The model under review builds one solid part; all positions refer to its coordinate system, in mm. A direction names the side the tool comes from. Coordinates: 2 decimals unless noted, no trailing zeros. Loops run counter-clockwise (first coordinate to the right, second up) from the corner with the lowest first, then second, coordinate; pieces in that order, holes last. Notation, with made-up numbers: (69, 55) - (105, 55) arc R38 ccw to (105, 94) - close; hole circle Ø2 at (21.25, -2). An arc over 180 degrees is marked (long way). Answer in a Markdown table with one row per item. Add a question column.
(1) Machinability: for faces 1 (the cylindrical face through (136.2, 0.9, 2.7)), 2 (the flat face through (76.637, 5, 6)), 3 (the cylindrical face through (136.25, 7.94, 2.72)), 4 (the flat face through (79.905, 4, 6)), which of the approach directions +Z, -Z, +X, -X, +Y, -Y give a long, thin tool a straight path to every point of the face, cutting with its end or side? Answer none if there is none.
(2) We need section A-A on z = 5.25. Write out the cut boundary in (x, y) (3 decimals).
(3) Mouldability with a two-part tool opening along Y and no side actions: class faces 5 (the cylindrical face through (0.95, 7.98, 1.93)), 6 (the flat face through (21, 5, 3.81)), 7 (the cylindrical face through (43.427, 4.185, 6.993)) as +Y half, -Y half, draft (parallel to the pull), parting line (faces both ways), or undercut.
(4) For P1, Ø5.5, axis at x = 127.5, y = 10.5, coming from the +Z side; P2, Ø6, axis at x = 109, y = 4.5, coming from the -Z side; P3, Ø0.5, axis at y = -0.5, z = 1, coming from the -X side; P4, Ø5.5, axis at x = 49.5, z = 5, coming from the +Y side, all flat-tipped, find the tip position at first contact; note any pin that passes through.
(5) For line 1 along X through (y, z) = (0.75, 4.25) (3 decimals); line 2 along Z through (x, y) = (24, 5.75); line 3 along Y through (x, z) = (75.5, 2.5), list the stretches that pass through material, from the lowest coordinate up.
(6) We need section C-C on x = 74.5. Write out the cut boundary in (y, z), plus the area to 3 significant figures.
(7) We need section D-D on y = 1.25. Write out the cut boundary in (x, z) (3 decimals).
(8) We need section B-B on y = 7.75. Write out the cut boundary in (x, z) (3 decimals).
Autodesk Inventor part; units mm, degrees
ref_plane "YZ Plane" through (0, 0, 0) normal (1, 0, 0) x (0, 1, 0)
ref_plane "XZ Plane" through (0, 0, 0) normal (0, 1, 0) x (-1, 0, 0)
ref_plane "XY Plane" through (0, 0, 0) normal (0, 0, 1) x (1, 0, 0)
sketch "Sketch1" plane through (0, 0, 0) normal (0, 0, 1) x (1, 0, 0)
  point P0 (0, 0)
sketch "Sketch2" plane through (0, 0, 0) normal (0, 0, 1) x (1, 0, 0)
  line L0 (0, 0) -> (137.16, 0)
  line L1 (137.16, 0) -> (137.16, 8.89)
  line L2 (137.16, 8.89) -> (0, 8.89)
  line L3 (0, 8.89) -> (0, 0)
  dimension "d0" = 137.16
  dimension "d3" = 8.89
extrude "Extrusion1" add sketch "Sketch2" along normal blind 3.81
sketch "Sketch3" plane through (0, 8.89, 0) normal (0, 1, 0) x (1, 0, 0)
  line L0 (137.16, 0) -> (137.16, -3.81)
  line L1 (137.16, 0) -> (119.5015, 0)
  line L2 (119.5015, 0) -> (119.5015, -1.6003)
  line L3 (119.5015, -1.6003) -> (137.16, -1.6003)
  line L4 (137.16, -1.6003) -> (137.16, 0)
  point P0 (0, 0)
extrude "Extrusion2" add sketch "Sketch3" along normal blind 3.81
sketch "Sketch4" plane through (0, 0, 0) normal (0, -1, 0) x (1, 0, 0)
  line L0 (0, 0) -> (137.16, 0)
  line L1 (119.5015, 1.6003) -> (137.16, 1.6003)
  line L2 (137.16, 0) -> (119.5015, 0)
  line L3 (119.5015, 0) -> (119.5015, 1.6003)
  line L4 (119.5015, 1.6003) -> (137.16, 1.6003)
  line L5 (137.16, 1.6003) -> (137.16, 0)
extrude "Extrusion3" add sketch "Sketch4" along normal blind 3.81
sketch "Sketch6" plane through (0, 0, 3.81) normal (0, 0, 1) x (1, 0, 0)
  line L0 (119.5015, 8.89) -> (0, 8.89)
  line L1 (0, 0) -> (119.5015, 0)
  line L2 (79.905, 8.89) -> (76.6366, 8.89)
  line L3 (76.6366, 8.89) -> (76.6366, 0)
  line L4 (76.6366, 0) -> (79.905, 0)
  line L5 (79.905, 0) -> (79.905, 8.89)
  dimension "d28" = 119.5015
extrude "Extrusion5" add sketch "Sketch6" along normal blind 7.62
sketch "Sketch7" plane through (79.905, 0, 3.81) normal (1, 0, 0) x (0, 0, -1)
  line L0 (-7.62, 0) -> (-7.62, 8.89)
  circle A0 centre (-7.62, 4.445) radius 4.445
  point P0 (3.81, 0)
extrude "Extrusion6" cut sketch "Sketch7" against normal blind 12.7
sketch "Sketch8" plane through (0, 0, 3.81) normal (0, 0, 1) x (1, 0, 0)
  line L0 (0, 0) -> (119.5015, 0)
  line L1 (119.5015, 8.89) -> (0, 8.89)
  line L2 (45.2172, 0) -> (41.5862, 0)
  line L3 (41.5862, 0) -> (41.5862, 8.89)
  line L4 (41.5862, 8.89) -> (45.2172, 8.89)
  line L5 (45.2172, 8.89) -> (45.2172, 0)
extrude "Extrusion7" add sketch "Sketch8" along normal blind 12.7
fillet "Fillet3" radius 3.175 8 edges at (0, 0, 1.905) (0, 8.89, 1.905) (137.16, 0, 2.7052) (137.16, 8.89, 2.7052) (137.16, -3.81, 0.8002) (137.16, 12.7, 0.8002) (119.5015, -3.81, 0.8002) (119.5015, 12.7, 0.8002)
extrude "Extrusion8" cut sketch "Sketch7" against normal through all
sketch "Sketch9" plane through (41.5862, 0, 16.51) normal (-1, 0, 0) x (0, 0, 1)
  circle A0 centre (-1.585, 4.5756) radius 5.8334
  point P0 (-16.51, 0)
extrude "Extrusion9" cut sketch "Sketch9" against normal through all
properties part number "stweet"
Outcome:
| question | item | result |
|---|---|---|
| 1 | face 1 | +Z, +X, -Y |
| 1 | face 2 | +Z, +Y, -Y |
| 1 | face 3 | +Z, +X, +Y |
| 1 | face 4 | +Z, +X, +Y, -Y |
| 2 | outline | (41.586, 0) - (45.217, 0) - (45.217, 8.89) - (41.586, 8.89) - close; (76.637, 0) - (79.905, 0) - (79.905, 8.89) - (76.637, 8.89) - close |
| 3 | face 5 | +Y half |
| 3 | face 6 | draft |
| 3 | face 7 | undercut |
| 4 | P1 | z = 3.81 |
| 4 | P2 | z = 0 |
| 4 | P3 | x = 119.5 |
| 4 | P4 | y = 8.89 |
| 5 | line 1 | 41.586 to 45.217, 76.637 to 79.905 |
| 5 | line 2 | 0 to 3.81 |
| 5 | line 3 | 0 to 8.89 |
| 6 | outline | (0, 0) - (8.89, 0) - (8.89, 3.81) - (0, 3.81) - close |
| 6 | area | 33.9 mm² |
| 7 | outline | (0.65, 0) - (137.16, 0) - (137.16, 1.6) - (136.51, 1.6) - (136.51, 3.81) - (79.905, 3.81) - (79.905, 8.34) - (76.637, 8.34) - (76.637, 3.81) - (45.217, 3.81) - (45.217, 8.34) - (41.586, 8.34) - (41.586, 3.81) - (0.65, 3.81) - close |
| 8 | outline | (0.738, 0) - (137.16, 0) - (137.16, 1.6) - (136.422, 1.6) - (136.422, 3.81) - (79.905, 3.81) - (79.905, 8.458) - (76.637, 8.458) - (76.637, 3.81) - (45.217, 3.81) - (45.217, 8.458) - (41.586, 8.458) - (41.586, 3.81) - (0.738, 3.81) - close |
